from build123d import *

# Parameters (mm, degrees)
BOSS_EXTRUDE1_DEPTH = 2.5
SKETCH16_R          = 2.225
CUT_EXTRUDE2_DEPTH  = 15


with BuildPart() as part:
    # Sketch1 → Boss-Extrude1 (new body)
    with BuildSketch(Plane.XY):
        with BuildLine():
            Line((3.125, -17.5), (3.125, -9.499177596))
            ThreePointArc((3.125, -9.499177596), (7.071067812, -7.071067812), (9.499177596, -3.125))
            Line((9.499177596, -3.125), (17.5, -3.125))
            ThreePointArc((17.5, -3.125), (19.5, 0), (17.5, 3.125))
            Line((17.5, 3.125), (9.499177596, 3.125))
            ThreePointArc((9.499177596, 3.125), (7.071067812, 7.071067812), (3.125, 9.499177596))
            Line((3.125, 9.499177596), (3.125, 17.5))
            ThreePointArc((3.125, 17.5), (0, 19.5), (-3.125, 17.5))
            Line((-3.125, 17.5), (-3.125, 9.499177596))
            ThreePointArc((-3.125, 9.499177596), (-7.071067812, 7.071067812), (-9.499177596, 3.125))
            Line((-9.499177596, 3.125), (-17.5, 3.125))
            ThreePointArc((-17.5, 3.125), (-19.5, 0), (-17.5, -3.125))
            Line((-17.5, -3.125), (-9.499177596, -3.125))
            ThreePointArc((-9.499177596, -3.125), (-7.071067812, -7.071067812), (-3.125, -9.499177596))
            Line((-3.125, -9.499177596), (-3.125, -17.5))
            ThreePointArc((-3.125, -17.5), (0, -19.5), (3.125, -17.5))
        make_face()
        with BuildLine():
            ThreePointArc((-9.868180698, -1.618335477), (-9.86763363, -1.621667831), (-9.867085436, -1.625))
            Line((-9.867085436, -1.625), (-9.878306468, -1.625))
            Line((-9.878306468, -1.625), (-17.120871128, -1.625))
            ThreePointArc((-17.120871128, -1.625), (-18, 0), (-17.120871128, 1.625))
            Line((-17.120871128, 1.625), (-9.878306468, 1.625))
            Line((-9.878306468, 1.625), (-9.867085436, 1.625))
            ThreePointArc((-9.867085436, 1.625), (-9.86763363, 1.621667831), (-9.868180698, 1.618335477))
            ThreePointArc((-9.868180698, 1.618335477), (-8.999177596, 0), (-9.868180698, -1.618335477))
        make_face(mode=Mode.SUBTRACT)
        with BuildLine():
            ThreePointArc((-1.618335477, -9.868180698), (0, -8.999177596), (1.618335477, -9.868180698))
            ThreePointArc((1.618335477, -9.868180698), (1.621667831, -9.86763363), (1.625, -9.867085436))
            Line((1.625, -9.867085436), (1.625, -9.878306468))
            Line((1.625, -9.878306468), (1.625, -17.120871128))
            ThreePointArc((1.625, -17.120871128), (0, -18), (-1.625, -17.120871128))
            Line((-1.625, -17.120871128), (-1.625, -9.878306468))
            Line((-1.625, -9.878306468), (-1.625, -9.867085436))
            ThreePointArc((-1.625, -9.867085436), (-1.621667831, -9.86763363), (-1.618335477, -9.868180698))
        make_face(mode=Mode.SUBTRACT)
        with BuildLine():
            Line((1.625, 9.878306468), (1.625, 9.867085436))
            ThreePointArc((1.625, 9.867085436), (1.621667831, 9.86763363), (1.618335477, 9.868180698))
            ThreePointArc((1.618335477, 9.868180698), (0, 8.999177596), (-1.618335477, 9.868180698))
            ThreePointArc((-1.618335477, 9.868180698), (-1.621667831, 9.86763363), (-1.625, 9.867085436))
            Line((-1.625, 9.867085436), (-1.625, 9.878306468))
            Line((-1.625, 9.878306468), (-1.625, 17.120871128))
            ThreePointArc((-1.625, 17.120871128), (0, 18), (1.625, 17.120871128))
            Line((1.625, 17.120871128), (1.625, 9.878306468))
        make_face(mode=Mode.SUBTRACT)
        with BuildLine():
            ThreePointArc((9.868180698, 1.618335477), (9.86763363, 1.621667831), (9.867085436, 1.625))
            Line((9.867085436, 1.625), (9.878306468, 1.625))
            Line((9.878306468, 1.625), (17.120871128, 1.625))
            ThreePointArc((17.120871128, 1.625), (18, 0), (17.120871128, -1.625))
            Line((17.120871128, -1.625), (9.878306468, -1.625))
            Line((9.878306468, -1.625), (9.867085436, -1.625))
            ThreePointArc((9.867085436, -1.625), (9.86763363, -1.621667831), (9.868180698, -1.618335477))
            ThreePointArc((9.868180698, -1.618335477), (8.999177596, 0), (9.868180698, 1.618335477))
        make_face(mode=Mode.SUBTRACT)
    extrude(amount=BOSS_EXTRUDE1_DEPTH)

    # Loft2: read off the stored shape, not the designer's step
    # Loft2: loft between two sections, ruled curve by curve
    loft2_from = [
        Edge.make_bspline([(3.048060313, 1.127753665, -15), (0.792552983, 7.223874291, -15), (-5.303567643, 4.968366961, -15), (-3.048060313, -1.127753665, -15), (-0.792552983, -7.223874291, -15), (5.303567643, -4.968366961, -15), (3.048060313, 1.127753665, -15)], [0, 0, 0, 0, 0.5, 0.5, 0.5, 1, 1, 1, 1], 3, [1, 0.333333333, 0.333333333, 1, 0.333333333, 0.333333333, 1]),
    ]
    loft2_to = [
        Edge.make_bspline([(4.41488096, 4.063105476, 0), (-3.711329991, 12.892867396, 0), (-12.541091911, 4.766656445, 0), (-4.41488096, -4.063105476, 0), (3.711329991, -12.892867396, 0), (12.541091911, -4.766656445, 0), (4.41488096, 4.063105476, 0)], [0, 0, 0, 0, 0.5, 0.5, 0.5, 1, 1, 1, 1], 3, [1, 0.333333333, 0.333333333, 1, 0.333333333, 0.333333333, 1]),
    ]
    loft2 = Solid(Shell([*[Face.make_surface_from_curves(loft2_from[k], loft2_to[k]) for k in range(1)], Face(Wire(loft2_from)), Face(Wire(loft2_to))]))
    add(loft2)

    # Sketch16 → Cut-Extrude2 (cut)
    with BuildSketch(Plane(origin=(0, 0, -15), x_dir=(-1, 0, 0), z_dir=(0, 0, -1))):
        Circle(SKETCH16_R)
    extrude(amount=-CUT_EXTRUDE2_DEPTH, mode=Mode.SUBTRACT)


solid = part.part
Read the model definition and answer for the solid it produces. Units are mm, in the model's axes. A direction names the side the tool comes from. Give positions to 0.01 mm unless a question says otherwise; leave off trailing zeros. Loops run counter-clockwise (first coordinate to the right, second up) from the corner with the lowest first, then second, coordinate; pieces in that order, holes last. Notation, with made-up numbers: (-27, -28) - (26, -28) arc R22 ccw to (26, 4) - close; hole circle Ø7 at (71, 45.25). An arc over 180 degrees is marked (long way). Answer as CSV lines item,"result". Start each with the question number.
1) Find section A-A (y = 12). Write down the section's boundary in (x, z) (3 decimals).
2) Find section C-C (y = 0). State how many separate pieces and enclosed holes the cut face has, then the cut area to 3 significant figures.
3) Which of the six approach directions +Z, -Z, +X, -X, +Y, -Y give full straight-line access (tool end or side, diameter ignored) to faces 1 (the face through (9, 0, 1)), 2 (the face through (7.02, -7.12, 1.23)), 3 (the face through (-3.125, -13, 1))?
4) Determine the mould class of faces 4 (the face through (1.625, 14, 1)), 5 (the face through (13, -3.125, 1)), 6 (the face through (-19.5, 0.1, 1.2)) for opening direction X: released by +X, released by -X, zero draft, split by the parting line, or undercut.
5) Each of these flat-tipped pins is pushed along its axis until it touches: pin 1 Ø1.2 at (y, z) = (-12.5, 1.5) entering from +X (3 decimals); pin 2 Ø1.2 at (x, z) = (14, 1.5) entering from -Y (3 decimals); pin 3 Ø1.2 at (x, z) = (-11.5, 1.5) entering from +Y (3 decimals); pin 4 Ø19.5 at (x, y) = (6.5, 4.5) entering from -Z. Where does it stop, or does it pass through?
Findings below:
1,outline,"(-3.125, 0) - (-1.625, 0) - (-1.625, 2.5) - (-3.125, 2.5) - close; (1.625, 0) - (3.125, 0) - (3.125, 2.5) - (1.625, 2.5) - close"
2,separate pieces,"3"
2,enclosed holes,"0"
2,area,"123 mm^2"
3,face 1,"+Z, -Z"
3,face 2,"+Z, -Z, +X, -Y"
3,face 3,"+Z, -Z, -X, -Y"
4,face 4,"undercut"
4,face 5,"zero draft"
4,face 6,"released by -X"
5,pin 1,"x = 3.125"
5,pin 2,"y = -3.125"
5,pin 3,"y = 3.125"
5,pin 4,"z = -15"
